Read the model definition and answer for the solid it produces. Units are mm, in the model's axes. Give positions to 0.01 mm unless a question says otherwise; leave off trailing zeros. Loops run counter-clockwise (first coordinate to the right, second up) from the corner with the lowest first, then second, coordinate; pieces in that order, holes last. Notation, with made-up numbers: (84, -37.75) - (103, -37.75) arc R11 ccw to (103, -23.75) - close; hole circle Ø9 at (37, 70). An arc over 180 degrees is marked (long way). Put each result on its own line as item: value. Start each with the question number.
1. A cutting plane is placed at C-C, the plane z = 1.35. Count the separate pieces of the cut face and the enclosed holes in it, plus the area to 3 significant figures.
2. A cutting plane is placed at B-B, the plane x = 198. Determine the outline of the cut face in (y, z).
3. Given pin 1 Ø0.9 at (y, z) = (-2, 1.5) entering from +X; pin 2 Ø0.9 at (x, z) = (2, 1) entering from +Y; pin 3 Ø0.9 at (x, z) = (223.5, 2) entering from -Y, each flat-ended and moving along its own axis, determine where each tip first touches the part or whether it passes through.
4. Consider L1, parallel to Y at x = 11, z = 0.6; L2, parallel to Y at x = 33, z = 1.8; L3, parallel to X at y = 34, z = 1.9. Determine where each line is inside the solid, lowest interval first. Write a range as from..to.
5. A cutting plane is placed at D-D, the plane y = 94. Determine the outline of the cut face in (x, z), plus the area to 3 significant figures.
6. A cutting plane is placed at A-A, the plane y = 29.5. Determine the outline of the cut face in (x, z), plus the area to 3 significant figures.
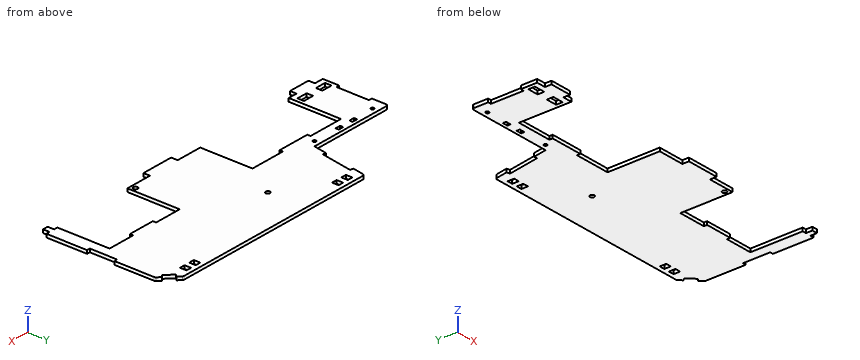
```python
from build123d import *

# Parameters (mm, degrees)
BOSS_EXTRUDE1_DEPTH     = 3
SKETCH2_R               = 2
CUT_EXTRUDE1_DEPTH      = 321.943920335
CUT_EXTRUDE2_DEPTH      = 321.943920335
CUT_EXTRUDE2_DEPTH_BACK = 321.943920335
SKETCH3_W               = 3
SKETCH3_H               = 30
SKETCH4_W               = 10
SKETCH4_H               = 6
CUT_EXTRUDE3_DEPTH      = 321.943920335
SKETCH5_R               = 1.5
SKETCH5_W               = 5
SKETCH5_H               = 3
CUT_EXTRUDE4_DEPTH      = 321.943920335
SKETCH6_W               = 5
SKETCH6_H               = 6
CUT_EXTRUDE5_DEPTH      = 321.943920335
FILLET1_R               = 2


with BuildPart() as part:
    # Sketch1 → Boss-Extrude1 (new body)
    with BuildSketch(Plane.XY):
        Polygon((0, 0), (8.5, 0), (8.5, -6), (28.5, -6), (28.5, 0), (37, 0), (37, 48), (70, 48), (70, 45), (100, 45), (100, 48), (133, 48), (133, 0), (157.5, 0), (157.5, -6), (187.5, -6), (187.5, 0), (212, 0), (212, 48), (237.5, 48), (237.5, 45), (262.5, 45), (262.5, 48), (288, 48), (288, 0), (291.5, 0), (291.5, -6), (296.5, -6), (296.5, 0), (300, 0), (300, 37.428932188), (297, 37.428932188), (297, 62.428932188), (300, 62.428932188), (300, 99.857864376), (296.464466094, 103.393398282), (294.343145751, 101.272077939), (287.272077939, 108.343145751), (289.393398282, 110.464466094), (285.857864376, 114), (89.521656958, 114), (80, 60), (0, 60), align=None)
    extrude(amount=BOSS_EXTRUDE1_DEPTH)

    # Sketch2 → Cut-Extrude1 (cut, through all)
    with BuildSketch(Plane(origin=(0, 0, 0), x_dir=(-1, 0, 0), z_dir=(0, 0, -1))):
        with Locations((-208, 4)):
            Circle(SKETCH2_R)
        with Locations((-153, 79)):
            Circle(SKETCH2_R)
    extrude(amount=-CUT_EXTRUDE1_DEPTH, mode=Mode.SUBTRACT)

    # Sketch3 → Cut-Extrude2 (cut, two sides: drawn at the far end of the back side and taken through both)
    with BuildSketch(Plane(origin=(0, 0, 0), x_dir=(-1, 0, 0), z_dir=(0, 0, -1)).offset(-CUT_EXTRUDE2_DEPTH_BACK)):
        Polygon((-87.40573319, 102), (-90.360156449, 101.479055467), (-85.150711119, 71.934822877), (-82.19628786, 72.45576741), align=None)
        with Locations((-1.5, 30)):
            Rectangle(SKETCH3_W, SKETCH3_H)
    extrude(amount=CUT_EXTRUDE2_DEPTH + CUT_EXTRUDE2_DEPTH_BACK, mode=Mode.SUBTRACT)

    # Sketch4 → Cut-Extrude3 (cut, through all)
    with BuildSketch(Plane(origin=(0, 0, 0), x_dir=(-1, 0, 0), z_dir=(0, 0, -1))):
        with Locations((-28.5, 8)):
            Rectangle(SKETCH4_W, SKETCH4_H)
        with Locations((-8.5, 8)):
            Rectangle(SKETCH4_W, SKETCH4_H)
    extrude(amount=-CUT_EXTRUDE3_DEPTH, mode=Mode.SUBTRACT)

    # Sketch5 → Cut-Extrude4 (cut, through all)
    with BuildSketch(Plane(origin=(0, 0, 0), x_dir=(-1, 0, 0), z_dir=(0, 0, -1))):
        with Locations((-11, 55)):
            Circle(SKETCH5_R)
        with Locations((-74, 55)):
            Circle(SKETCH5_R)
        with Locations((-47.5, 55.5)):
            Rectangle(SKETCH5_W, SKETCH5_H)
        with Locations((-32.5, 55.5)):
            Rectangle(SKETCH5_W, SKETCH5_H)
    extrude(amount=-CUT_EXTRUDE4_DEPTH, mode=Mode.SUBTRACT)

    # Sketch6 → Cut-Extrude5 (cut, through all)
    with BuildSketch(Plane(origin=(0, 0, 0), x_dir=(-1, 0, 0), z_dir=(0, 0, -1))):
        with Locations((-275.357864376, 107)):
            Rectangle(SKETCH6_W, SKETCH6_H)
        with Locations((-265.357864376, 107)):
            Rectangle(SKETCH6_W, SKETCH6_H)
        with Locations((-110.357864376, 107)):
            Rectangle(SKETCH6_W, SKETCH6_H)
        with Locations((-100.357864376, 107)):
            Rectangle(SKETCH6_W, SKETCH6_H)
    extrude(amount=-CUT_EXTRUDE5_DEPTH, mode=Mode.SUBTRACT)

    # Fillet1
    fillet1_edges = [part.edges().sort_by_distance(p)[0] for p in [
        (0, 60, 1.5),
        (89.521656958, 114, 1.5),
        (285.857864376, 114, 1.5),
        (300, 99.857864376, 1.5),
    ]]
    fillet(fillet1_edges, radius=FILLET1_R)


solid = part.part
```
Return value:
1. separate pieces: 1
1. enclosed holes: 12
1. area: 21,200 mm2
2. outline: (0, 0) - (114, 0) - (114, 3) - (0, 3) - close
3. pin 1: stops at x = 296.5
3. pin 2: stops at y = 60
3. pin 3: stops at y = 48
4. L1: y = -6..5, 11..53.5, 56.5..60
4. L2: y = 0..5, 11..54, 57..60
4. L3: x = 3..37, 133..212, 288..300
5. outline: (89.04, 0) - (300, 0) - (300, 3) - (89.04, 3) - close
5. area: 633 mm2
6. outline: (3, 0) - (37, 0) - (37, 3) - (3, 3) - close; (133, 0) - (212, 0) - (212, 3) - (133, 3) - close; (288, 0) - (300, 0) - (300, 3) - (288, 3) - close
6. area: 375 mm2
